```python
from build123d import *

# Parameters (mm, degrees)
SKIZZE1_W                       = 14.25
SKIZZE1_H                       = 14.25
AUFSATZ_LINEAR_AUSTRAGEN1_DEPTH = 16
FASE1_SIZE                      = 4.1
VERRUNDUNG2_R                   = 0.5
VERRUNDUNG3_R                   = 0.25
VERRUNDUNG4_R                   = 0.25


with BuildPart() as part:
    # Skizze1 → Aufsatz-Linear austragen1 (new body)
    with BuildSketch(Plane(origin=(0, 0, 0), x_dir=(1, 0, 0), z_dir=(0, 1, 0))):
        Rectangle(SKIZZE1_W, SKIZZE1_H)
    extrude(amount=AUFSATZ_LINEAR_AUSTRAGEN1_DEPTH)

    # Skizze6 → Schnitt-Rotation4 (revolve, cut)
    with BuildSketch(Plane(origin=(0, 0, 0), x_dir=(0, 0, -1), z_dir=(1, 0, 0))):
        Polygon((6.25, 16), (13.25, 16), (13.25, 9), (4, 9), (4, 13), (6.25, 13), align=None)
    revolve(axis=Axis((0, 0, 0), (0, 1, 0)), mode=Mode.SUBTRACT)

    # Fase1
    # the kernel refuses this chamfer: 4.1 mm, written as the material it takes off along each edge
    with BuildSketch(Plane(origin=(17.668900251, 9, 7.125), x_dir=(0, 0.027495876610586303, -0.9996219169112966), z_dir=(-1, 0, 0))) as fase1_piece_1_section:
        Polygon((FASE1_SIZE * 0.999621916911, FASE1_SIZE * 0.0274958766106), (-FASE1_SIZE * 0.0274958766106, FASE1_SIZE * 0.999621916911), (0, 0), align=None)
    fase1_piece_1 = extrude(amount=35.337800501, mode=Mode.PRIVATE)
    fase1_piece_1 = fase1_piece_1 - Plane(origin=(0, 7.640449018, 0), x_dir=(0, 0, -1), z_dir=(0, 1, 0)) * Cylinder(4, 88, mode=Mode.PRIVATE)
    add(fase1_piece_1, mode=Mode.SUBTRACT)
    with BuildSketch(Plane(origin=(7.125, 9, -17.668900251), x_dir=(0.027495876610586303, -0.9996219169112966, 0), z_dir=(0, 0, 1))) as fase1_piece_2_section:
        Polygon((FASE1_SIZE * 0.999621916911, -FASE1_SIZE * 0.0274958766106), (-FASE1_SIZE * 0.0274958766106, -FASE1_SIZE * 0.999621916911), (0, 0), align=None)
    fase1_piece_2 = extrude(amount=35.337800501, mode=Mode.PRIVATE)
    fase1_piece_2 = fase1_piece_2 - Plane(origin=(0, 7.640449013, 0), x_dir=(0, 0, -1), z_dir=(0, 1, 0)) * Cylinder(4, 88, mode=Mode.PRIVATE)
    add(fase1_piece_2, mode=Mode.SUBTRACT)
    with BuildSketch(Plane(origin=(-17.668900251, 9, -7.125), x_dir=(0, -0.9996219169112966, -0.027495876610586303), z_dir=(1, 0, 0))) as fase1_piece_3_section:
        Polygon((FASE1_SIZE * 0.999621916911, -FASE1_SIZE * 0.0274958766106), (-FASE1_SIZE * 0.0274958766106, -FASE1_SIZE * 0.999621916911), (0, 0), align=None)
    fase1_piece_3 = extrude(amount=35.337800501, mode=Mode.PRIVATE)
    fase1_piece_3 = fase1_piece_3 - Plane(origin=(0, 7.640449014, 0), x_dir=(0, 0, -1), z_dir=(0, 1, 0)) * Cylinder(4, 88, mode=Mode.PRIVATE)
    add(fase1_piece_3, mode=Mode.SUBTRACT)
    with BuildSketch(Plane(origin=(-7.125, 9, 17.668900251), x_dir=(0.9996219169112966, 0.027495876610586303, 0), z_dir=(0, 0, -1))) as fase1_piece_4_section:
        Polygon((FASE1_SIZE * 0.999621916911, FASE1_SIZE * 0.0274958766106), (-FASE1_SIZE * 0.0274958766106, FASE1_SIZE * 0.999621916911), (0, 0), align=None)
    fase1_piece_4 = extrude(amount=35.337800501, mode=Mode.PRIVATE)
    fase1_piece_4 = fase1_piece_4 - Plane(origin=(0, 7.640449018, 0), x_dir=(0, 0, -1), z_dir=(0, 1, 0)) * Cylinder(4, 88, mode=Mode.PRIVATE)
    add(fase1_piece_4, mode=Mode.SUBTRACT)

    # Verrundung2
    verrundung2_edges = [part.edges().sort_by_distance(p)[0] for p in [
        (0, 16, 6.25),
    ]]
    fillet(verrundung2_edges, radius=VERRUNDUNG2_R)

    # Verrundung3
    verrundung3_edges = [part.edges().sort_by_distance(p)[0] for p in [
        (-7.125, 4.9, 0),
        (0, 4.9, -7.125),
        (7.125, 4.9, 0),
        (0, 4.9, 7.125),
    ]]
    fillet(verrundung3_edges, radius=VERRUNDUNG3_R)

    # Verrundung4
    verrundung4_edges = [part.edges().sort_by_distance(p)[0] for p in [
        (0, 13, 6.25),
    ]]
    fillet(verrundung4_edges, radius=VERRUNDUNG4_R)


solid = part.part
```
Could you check a few things on this model? Use its own coordinates, in mm. A direction names the side the tool comes from. Round coordinates to 2 decimals unless told otherwise and drop trailing zeros. Order: outer loops, then holes, each group sorted by start corner. A loop starts at its lowest first (then second) coordinate and runs counter-clockwise, first axis right, second up. Notation, with made-up numbers: M 17,83.5 L 39,83.5 A35 cw 39,118.5 Z; hole C 67.25,72.5 d2. An arc over 180 degrees is marked long. One line per question, with ' | ' between items. Start each with the question number.
(1) Thinking about a two-plate mould opening in Y: for faces 4 (the face through (0, 16, 0)), 5 (the face through (-0.099, 6.511, -5.514)), 6 (the face through (0, 2, 7.125)), which applies, +Y half, -Y half, draft (parallel to the pull), parting line (faces both ways), or undercut?
(2) Please list where these lines run through material, in increasing order: line 1 along Y through (x, z) = (-1, -4) (3 decimals); line 2 along Y through (x, z) = (4.5, 1.25) (3 decimals); line 3 along X through (y, z) = (14.5, -4.25).
(3) For faces 1 (the face through (-1.88, 14.39, -5.96)), 2 (the face through (-1.09, 10.47, -3.85)), 3 (the face through (0, 2, -7.125)), which set-ups out of +Z, -Z, +X, -X, +Y, -Y let a thin tool reach every point of the face, with its end or its side?
(4) Suppose I cut it at B-B on z = 0. List the corners of the cut face in (x, y) for me (3 decimals).
(5) Suppose I cut it at C-C on y = 14.75. List the corners of the cut face in (x, z) for me, then the cut area to 3 significant figures.
(6) For P1, Ø4, axis at y = 5.5, z = 3, coming from the +X side (3 decimals); P2, Ø5, axis at y = 10, z = 2, coming from the -X side (3 decimals); P3, Ø1, axis at y = 9.5, z = 3, coming from the +X side; P4, Ø8, axis at x = 3, y = 12.5, coming from the +Z side, each with a flat end and sliding along its axis, tell me the tip position at first contact or that it passes through.
(7) Suppose I cut it at D-D on y = 10.25. List the corners of the cut face in (x, z) for me, then the cut area to 3 significant figures.
(8) Suppose I cut it at A-A on x = 0. List the corners of the cut face in (y, z) for me (3 decimals), then the cut area to 3 significant figures.
Geometry results:
1) face 4: +Y half | face 5: undercut | face 6: draft
2) line 1: 0 to 8.025, 13 to 16 | line 2: 0 to 7.525, 13 to 16 | line 3: -4.58 to 4.58
3) face 1: +Y | face 2: none | face 3: -Z, +X, -X, +Y, -Y
4) outline: M -7.125,0 L 7.125,0 L 7.125,4.796 A0.25 ccw 7.052,4.973 L 4,8.025 L 4,13 L 6,13 A0.25 ccw 6.25,13.25 L 6.25,15.5 A0.5 ccw 5.75,16 L -5.75,16 A0.5 ccw -6.25,15.5 L -6.25,13.25 A0.25 ccw -6,13 L -4,13 L -4,8.025 L -7.052,4.973 A0.25 ccw -7.125,4.796 Z
5) outline: C 0,0 d12.5 | area: 123 mm²
6) P1: x = 7.125 | P2: x = -4.525 | P3: x = 3.12 | P4: z = 6.25
7) outline: C 0,0 d8 | area: 50.3 mm²
8) outline: M 0,-7.125 L 4.796,-7.125 A0.25 ccw 4.973,-7.052 L 8.025,-4 L 13,-4 L 13,-6 A0.25 ccw 13.25,-6.25 L 15.5,-6.25 A0.5 ccw 16,-5.75 L 16,5.75 A0.5 ccw 15.5,6.25 L 13.25,6.25 A0.25 ccw 13,6 L 13,4 L 8.025,4 L 4.973,7.052 A0.25 ccw 4.796,7.125 L 0,7.125 Z | area: 182 mm²
